Build history of the part. All positions in model axes, mm. Face numbers are marked on the shaded views. A direction names the side the tool comes from. Round coordinates to 2 decimals unless told otherwise and drop trailing zeros. Loops run counter-clockwise (first coordinate to the right, second up) from the corner with the lowest first, then second, coordinate; pieces in that order, holes last. Notation, with made-up numbers: (83.25, 26) -> (111.25, 26) arc R24 ccw to (111.25, 53) -> close; hole circle Ø1 at (-21.5, 16). An arc over 180 degrees is marked (long way). Put each result on its own line as item: value. Start each with the question number.
Item 1: Cut at A-A, the plane y = 33. List the corners of the cut face in (x, z) (3 decimals), plus the area to 3 significant figures.
Item 2: Cut at B-B, the plane x = 0. List the corners of the cut face in (y, z) (3 decimals), plus the area to 3 significant figures.
Item 3: Drill centre lines: probe 1 along Y at (x, z) = (9.5, -19); probe 2 along Y at (x, z) = (-4, 16.5); probe 3 along X at (y, z) = (28.5, 7) (3 decimals). Where is each one in solid material? Low to high. Write a range as [from, to].
Item 4: Tool access for the marked faces 1, 2, 3 and 4: list every direction of +Z, -Z, +X, -X, +Y, -Y with a clear straight run to the whole face (end or side of a thin tool).
Item 5: Cut at C-C, the plane z = 0. List the corners of the cut face in (x, y) (3 decimals), plus the area to 3 significant figures.
Item 6: Cut at D-D, the plane z = -11.5. List the corners of the cut face in (x, y) (3 decimals), plus the area to 3 significant figures.
Item 7: Flat gauge pins, fed straight in: pin 1 Ø1.6 at (x, y) = (-24, 46) entering from -Z; pin 2 Ø3 at (x, z) = (23.622, -23.622) entering from +Y; pin 3 Ø3.5 at (y, z) = (55, 25) entering from -X; pin 4 Ø1.5 at (x, z) = (17, 21.5) entering from -Y. Where does each tip first touch, or does it go through?
```python
from build123d import *

# Parameters (mm, degrees)
SKETCH1_R           = 2.54
BOSS_EXTRUDE1_DEPTH = 4.699
BOSS_EXTRUDE2_DEPTH = 72.771
FILLET1_R           = 3.81
FILLET2_R           = 2.54
FILLET3_R           = 1.27
SKETCH3_R           = 19.05
BOSS_EXTRUDE3_DEPTH = 1.524
CUT_EXTRUDE1_START  = -6.35
SKETCH5_R           = 22.225
CUT_EXTRUDE1_DEPTH  = 66.802
SKETCH4_R           = 3.175
CUT_EXTRUDE4_DEPTH  = 12.7


with BuildPart() as part:
    # Sketch1 → Boss-Extrude1 (new body)
    with BuildSketch(Plane(origin=(0, 0, 0), x_dir=(1, 0, 0), z_dir=(0, 1, 0))):
        with BuildLine():
            Line((-23.622, 28.575), (23.622, 28.575))
            ThreePointArc((23.622, 28.575), (27.124299887, 27.124299887), (28.575, 23.622))
            Line((28.575, 23.622), (28.575, -23.622))
            ThreePointArc((28.575, -23.622), (27.124299887, -27.124299887), (23.622, -28.575))
            Line((23.622, -28.575), (-23.622, -28.575))
            ThreePointArc((-23.622, -28.575), (-27.124299887, -27.124299887), (-28.575, -23.622))
            Line((-28.575, -23.622), (-28.575, 23.622))
            ThreePointArc((-28.575, 23.622), (-27.124299887, 27.124299887), (-23.622, 28.575))
        make_face()
        with Locations(Location((-23.622, 23.622, 0), (0, 0, 270))):
            Circle(SKETCH1_R, mode=Mode.SUBTRACT)
        with Locations(Location((23.622, 23.622, 0), (0, 0, 270))):
            Circle(SKETCH1_R, mode=Mode.SUBTRACT)
        with Locations(Location((23.622, -23.622, 0), (0, 0, 270))):
            Circle(SKETCH1_R, mode=Mode.SUBTRACT)
        with Locations(Location((-23.622, -23.622, 0), (0, 0, 270))):
            Circle(SKETCH1_R, mode=Mode.SUBTRACT)
    extrude(amount=BOSS_EXTRUDE1_DEPTH)

    # Sketch2 → Boss-Extrude2 (add)
    with BuildSketch(Plane(origin=(0, 4.699, 0), x_dir=(1, 0, 0), z_dir=(0, 1, 0))):
        Polygon((-19.05, -28.575), (-19.05, -19.05), (-28.575, -19.05), (-28.575, 19.05), (-19.05, 19.05), (-19.05, 28.575), (19.05, 28.575), (19.05, 19.05), (28.575, 19.05), (28.575, -19.05), (19.05, -19.05), (19.05, -28.575), align=None)
    extrude(amount=BOSS_EXTRUDE2_DEPTH)

    # Fillet1
    fillet1_edges = [part.edges().sort_by_distance(p)[0] for p in [
        (-19.05, 41.0845, 19.05),
        (-19.05, 41.0845, -19.05),
        (19.05, 41.0845, -19.05),
        (19.05, 41.0845, 19.05),
    ]]
    fillet(fillet1_edges, radius=FILLET1_R)

    # Fillet2
    fillet2_edges = [part.edges().sort_by_distance(p)[0] for p in [
        (28.575, 41.0845, -19.05),
        (19.05, 41.0845, -28.575),
        (28.575, 41.0845, 19.05),
        (-19.05, 41.0845, -28.575),
        (-28.575, 41.0845, -19.05),
        (-19.05, 41.0845, 28.575),
        (-28.575, 41.0845, 19.05),
        (19.05, 41.0845, 28.575),
    ]]
    fillet(fillet2_edges, radius=FILLET2_R)

    # Fillet3
    fillet3_edges = [part.edges().sort_by_distance(p)[0] for p in [
        (24.4475, 77.47, -19.05),
        (28.575, 77.47, 0),
        (0, 77.47, 28.575),
        (19.05, 77.47, 24.4475),
        (0, 77.47, -28.575),
        (-19.05, 77.47, -24.4475),
        (-28.575, 77.47, 0),
        (-24.4475, 77.47, 19.05),
        (18.306051224, 77.47, 27.831051224),
        (-27.831051224, 77.47, 18.306051224),
        (-18.306051224, 77.47, 27.831051224),
        (-27.831051224, 77.47, -18.306051224),
        (-18.306051224, 77.47, -27.831051224),
        (27.831051224, 77.47, 18.306051224),
        (18.306051224, 77.47, -27.831051224),
        (27.831051224, 77.47, -18.306051224),
        (-19.05, 77.47, 24.4475),
        (-24.4475, 77.47, -19.05),
        (19.05, 77.47, -24.4475),
        (24.4475, 77.47, 19.05),
        (-20.165923164, 77.47, 20.165923164),
        (-20.165923164, 77.47, -20.165923164),
        (20.165923164, 77.47, -20.165923164),
        (20.165923164, 77.47, 20.165923164),
    ]]
    fillet(fillet3_edges, radius=FILLET3_R)

    # Sketch3 → Boss-Extrude3 (add)
    with BuildSketch(Plane.XZ):
        with Locations(Location((0, 0, 0), (0, 0, 90))):
            Circle(SKETCH3_R)
    extrude(amount=BOSS_EXTRUDE3_DEPTH)

    # Sketch5 → Cut-Extrude1 (cut)
    with BuildSketch(Plane.XZ.offset(CUT_EXTRUDE1_START)):
        with Locations(Location((0, 0, 0), (0, 0, 270))):
            Circle(SKETCH5_R)
    extrude(amount=-CUT_EXTRUDE1_DEPTH, mode=Mode.SUBTRACT)

    # Sketch4 → Cut-Extrude4 (cut)
    with BuildSketch(Plane.XZ.offset(1.524)):
        with Locations(Location((0, 0, 0), (0, 0, 270))):
            Circle(SKETCH4_R)
    extrude(amount=-CUT_EXTRUDE4_DEPTH, mode=Mode.SUBTRACT)


solid = part.part
```
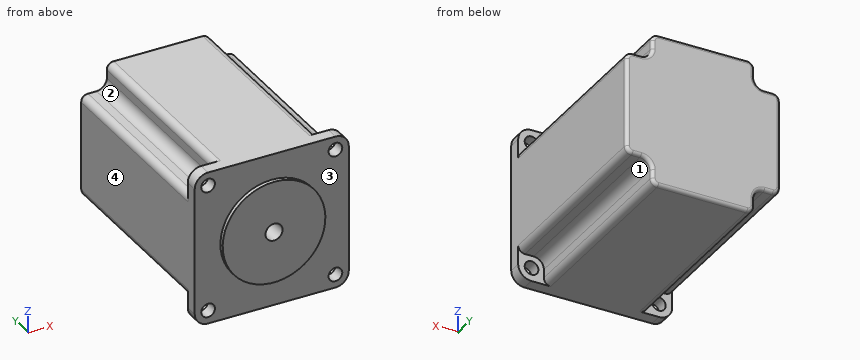
Reply:
1. outline: (-28.575, -16.51) arc R2.54 ccw to (-26.035, -19.05) -> (-22.86, -19.05) arc R3.81 cw to (-19.05, -22.86) -> (-19.05, -26.035) arc R2.54 ccw to (-16.51, -28.575) -> (16.51, -28.575) arc R2.54 ccw to (19.05, -26.035) -> (19.05, -22.86) arc R3.81 cw to (22.86, -19.05) -> (26.035, -19.05) arc R2.54 ccw to (28.575, -16.51) -> (28.575, 16.51) arc R2.54 ccw to (26.035, 19.05) -> (22.86, 19.05) arc R3.81 cw to (19.05, 22.86) -> (19.05, 26.035) arc R2.54 ccw to (16.51, 28.575) -> (-16.51, 28.575) arc R2.54 ccw to (-19.05, 26.035) -> (-19.05, 22.86) arc R3.81 cw to (-22.86, 19.05) -> (-26.035, 19.05) arc R2.54 ccw to (-28.575, 16.51) -> close; hole circle Ø44.45 at (0, 0)
1. area: 1,350 mm^2
2. outline: (-1.524, -19.05) -> (0, -19.05) -> (0, -28.575) -> (76.2, -28.575) arc R1.27 ccw to (77.47, -27.305) -> (77.47, 27.305) arc R1.27 ccw to (76.2, 28.575) -> (0, 28.575) -> (0, 19.05) -> (-1.524, 19.05) -> (-1.524, 3.175) -> (6.35, 3.175) -> (6.35, 22.225) -> (73.152, 22.225) -> (73.152, -22.225) -> (6.35, -22.225) -> (6.35, -3.175) -> (-1.524, -3.175) -> close
2. area: 1,470 mm^2
3. probe 1: y = [0, 6.35], [73.15, 77.47]
3. probe 2: y = [-1.52, 6.35], [73.15, 77.47]
3. probe 3: x = [-28.575, -21.094], [21.094, 28.575]
4. face 1: -Z, +X, +Y
4. face 2: +Z, -X, +Y
4. face 3: -Y
4. face 4: +Z, -Z, -X, +Y, -Y
5. outline: (-28.575, 0) -> (-19.05, 0) -> (-19.05, -1.524) -> (-3.175, -1.524) -> (-3.175, 6.35) -> (-22.225, 6.35) -> (-22.225, 73.152) -> (22.225, 73.152) -> (22.225, 6.35) -> (3.175, 6.35) -> (3.175, -1.524) -> (19.05, -1.524) -> (19.05, 0) -> (28.575, 0) -> (28.575, 76.2) arc R1.27 ccw to (27.305, 77.47) -> (-27.305, 77.47) arc R1.27 ccw to (-28.575, 76.2) -> close
5. area: 1,470 mm^2
6. outline: (-28.575, 0) -> (-15.187, 0) -> (-15.187, -1.524) -> (15.187, -1.524) -> (15.187, 0) -> (28.575, 0) -> (28.575, 76.2) arc R1.27 ccw to (27.305, 77.47) -> (-27.305, 77.47) arc R1.27 ccw to (-28.575, 76.2) -> close; hole (-19.018, 6.35) -> (19.018, 6.35) -> (19.018, 73.152) -> (-19.018, 73.152) -> close
6. area: 1,930 mm^2
7. pin 1: stops at z = -19.05
7. pin 2: passes through
7. pin 3: stops at x = -19.05
7. pin 4: stops at y = 0
